The listing builds one solid part. Answer for the finished solid, in the listing's coordinates (mm). A direction names the side the tool comes from. Round coordinates to 2 decimals unless told otherwise and drop trailing zeros. Write each loop counter-clockwise with the first axis right and the second up, starting at its lowest first coordinate (ties: lowest second). Pieces come first, ordered by that corner, then holes.
Item 1: A tool of negligible diameter and unlimited length cuts with its end or side. For faces 4 (the face through (143, 15, -7)), 5 (the face through (70.499, -19.205, 0.877)), from which of +Z, -Z, +X, -X, +Y, -Y can it reach the whole face along a straight path? Write none if from no direction.
Item 2: Find section C-C on x = 97.5. Give the vertices of the cut face in (y, z), then the cut area to 3 significant figures.
Item 3: Find section A-A on y = 0. Give the vertices of the cut face in (x, z).
Item 4: Find section B-B on z = 2.5. Give the vertices of the cut face in (x, y).
Item 5: For a pull along Y with two mould halves and no side action, classify faces 1 (the face through (70.499, -18.256, 10.378)), 2 (the face through (70.499, -19.961, -10.382)), 3 (the face through (0, 15, -7)) as +Y half, -Y half, draft (parallel to the pull), parting line (faces both ways), or undercut.
Item 6: Find the intervals of material crossed by probe 1 along Z at (x, y) = (41.5, -1); probe 2 along Y at (x, z) = (111.5, 0); probe 3 along Z at (x, y) = (111.5, 7.5), in increasing order.
Item 7: Each of these flat-tipped pins is pushed along its axis until it touches: pin 1 (1 mm diameter, centred on x = 20, z = 7, fed in from +Y); pin 2 (8 mm diameter, centred on x = 116, z = 17, fed in from +Y); pin 3 (10 mm diameter, centred on x = 73, y = 12.5, fed in from -Z). Where does it stop, or does it pass through?
```python
from build123d import *

# Parameters (mm, degrees)
SKETCH1_R           = 22.5
SKETCH1_R_2         = 16
BOSS_EXTRUDE1_DEPTH = 143


with BuildPart() as part:
    # Sketch1 → Boss-Extrude1 (new body)
    with BuildSketch(Plane(origin=(0, 0, 0), x_dir=(0, 0, -1), z_dir=(1, 0, 0))):
        Circle(SKETCH1_R)
        with BuildLine():
            ThreePointArc((0.798223616, -17.481785923), (8.75, -15.155444566), (14.740558905, -9.432174891))
            Line((14.740558905, -9.432174891), (17.688670686, -11.318609869))
            ThreePointArc((17.688670686, -11.318609869), (10.5, -18.186533479), (0.95786834, -20.978143108))
            Line((0.95786834, -20.978143108), (0.798223616, -17.481785923))
        make_face(mode=Mode.SUBTRACT)
        with BuildLine():
            Line((18.646539025, -9.659533238), (15.538782521, -8.049611032))
            ThreePointArc((15.538782521, -8.049611032), (17.5, 0), (15.538782521, 8.049611032))
            Line((15.538782521, 8.049611032), (18.646539025, 9.659533238))
            ThreePointArc((18.646539025, 9.659533238), (21, 0), (18.646539025, -9.659533238))
        make_face(mode=Mode.SUBTRACT)
        with BuildLine():
            Line((-0.798223616, -17.481785923), (-0.95786834, -20.978143108))
            ThreePointArc((-0.95786834, -20.978143108), (-10.5, -18.186533479), (-17.688670686, -11.318609869))
            Line((-17.688670686, -11.318609869), (-14.740558905, -9.432174891))
            ThreePointArc((-14.740558905, -9.432174891), (-8.75, -15.155444566), (-0.798223616, -17.481785923))
        make_face(mode=Mode.SUBTRACT)
        with BuildLine():
            Line((17.688670686, 11.318609869), (14.740558905, 9.432174891))
            ThreePointArc((14.740558905, 9.432174891), (8.75, 15.155444566), (0.798223616, 17.481785923))
            Line((0.798223616, 17.481785923), (0.95786834, 20.978143108))
            ThreePointArc((0.95786834, 20.978143108), (10.5, 18.186533479), (17.688670686, 11.318609869))
        make_face(mode=Mode.SUBTRACT)
        with BuildLine():
            Line((-15.538782521, -8.049611032), (-18.646539025, -9.659533238))
            ThreePointArc((-18.646539025, -9.659533238), (-21, 0), (-18.646539025, 9.659533238))
            Line((-18.646539025, 9.659533238), (-15.538782521, 8.049611032))
            ThreePointArc((-15.538782521, 8.049611032), (-17.5, 0), (-15.538782521, -8.049611032))
        make_face(mode=Mode.SUBTRACT)
        with BuildLine():
            Line((-0.95786834, 20.978143108), (-0.798223616, 17.481785923))
            ThreePointArc((-0.798223616, 17.481785923), (-8.75, 15.155444566), (-14.740558905, 9.432174891))
            Line((-14.740558905, 9.432174891), (-17.688670686, 11.318609869))
            ThreePointArc((-17.688670686, 11.318609869), (-10.5, 18.186533479), (-0.95786834, 20.978143108))
        make_face(mode=Mode.SUBTRACT)
        Circle(SKETCH1_R_2, mode=Mode.SUBTRACT)
    extrude(amount=BOSS_EXTRUDE1_DEPTH)


solid = part.part
```
Check values:
1. face 4: +Z, -Z, +X, +Y, -Y
1. face 5: +X, -X
2. outline: circle Ø45 at (0, 0); hole (-20.98, -0.96) arc R21 ccw to (-11.32, -17.69) - (-9.43, -14.74) arc R17.5 cw to (-17.48, -0.8) - close; hole (-20.98, 0.96) - (-17.48, 0.8) arc R17.5 cw to (-9.43, 14.74) - (-11.32, 17.69) arc R21 ccw to start; hole circle Ø32 at (0, 0); hole (-9.66, -18.65) arc R21 ccw to (9.66, -18.65) - (8.05, -15.54) arc R17.5 cw to (-8.05, -15.54) - close; hole (-9.66, 18.65) - (-8.05, 15.54) arc R17.5 cw to (8.05, 15.54) - (9.66, 18.65) arc R21 ccw to start; hole (9.43, -14.74) - (11.32, -17.69) arc R21 ccw to (20.98, -0.96) - (17.48, -0.8) arc R17.5 cw to start; hole (9.43, 14.74) arc R17.5 cw to (17.48, 0.8) - (20.98, 0.96) arc R21 ccw to (11.32, 17.69) - close
2. area: 400 mm2
3. outline: (0, -22.5) - (143, -22.5) - (143, -21) - (0, -21) - close; (0, -17.5) - (143, -17.5) - (143, -16) - (0, -16) - close; (0, 16) - (143, 16) - (143, 17.5) - (0, 17.5) - close; (0, 21) - (143, 21) - (143, 22.5) - (0, 22.5) - close
4. outline: (0, -22.36) - (143, -22.36) - (143, -20.85) - (0, -20.85) - close; (0, -17.32) - (143, -17.32) - (143, -15.8) - (0, -15.8) - close; (0, 15.8) - (143, 15.8) - (143, 17.32) - (0, 17.32) - close; (0, 20.85) - (143, 20.85) - (143, 22.36) - (0, 22.36) - close
5. face 1: undercut
5. face 2: parting line
5. face 3: draft
6. probe 1: z = -22.48 to -20.98, -17.47 to -15.97, 15.97 to 17.47, 20.98 to 22.48
6. probe 2: y = -22.5 to -16, 16 to 22.5
6. probe 3: z = -21.21 to -19.62, -15.81 to -14.13, 14.13 to 15.81, 19.62 to 21.21
7. pin 1: stops at y = 21.54
7. pin 2: stops at y = 18.36
7. pin 3: stops at z = -21.21
